Build history of the part. All positions in model axes, mm. Give positions to 0.01 mm unless a question says otherwise; leave off trailing zeros. Write each loop counter-clockwise with the first axis right and the second up, starting at its lowest first coordinate (ties: lowest second). Pieces come first, ordered by that corner, then holes. Notation, with made-up numbers: (57, 60.5) - (89, 60.5) arc R18 cw to (89, 84.5) - close; hole circle Ø4 at (-26.75, 77.5). An arc over 180 degrees is marked (long way). Use one line per item in the form item = value. Start each with the question number.
from build123d import *

# Parameters (mm, degrees)
F1_DEPTH = 400
F3_DEPTH = 25.001
F4_R     = 7.9375
F5_DEPTH = 25.001


with BuildPart() as f1:
    # F0 (on Top) → F1 (new body)
    with BuildSketch(Plane.XY):
        with BuildLine():
            ThreePointArc((12.5, 9.5), (11.62132, 11.62132), (9.5, 12.5))
            Line((9.5, 12.5), (-9.5, 12.5))
            ThreePointArc((-9.5, 12.5), (-11.62132, 11.62132), (-12.5, 9.5))
            Line((-12.5, 9.5), (-12.5, -9.5))
            ThreePointArc((-12.5, -9.5), (-11.62132, -11.62132), (-9.5, -12.5))
            Line((-9.5, -12.5), (9.5, -12.5))
            ThreePointArc((9.5, -12.5), (11.62132, -11.62132), (12.5, -9.5))
            Line((12.5, -9.5), (12.5, 9.5))
        make_face()
        with BuildLine():
            Line((-6.5, 9.5), (6.5, 9.5))
            ThreePointArc((6.5, 9.5), (8.62132, 8.62132), (9.5, 6.5))
            Line((9.5, 6.5), (9.5, -6.5))
            ThreePointArc((9.5, -6.5), (8.62132, -8.62132), (6.5, -9.5))
            Line((6.5, -9.5), (-6.5, -9.5))
            ThreePointArc((-6.5, -9.5), (-8.62132, -8.62132), (-9.5, -6.5))
            Line((-9.5, -6.5), (-9.5, 6.5))
            ThreePointArc((-9.5, 6.5), (-8.62132, 8.62132), (-6.5, 9.5))
        make_face(mode=Mode.SUBTRACT)
    extrude(amount=F1_DEPTH)

    # F2 (on face) → F3 (cut, through all)
    with BuildSketch(Plane(origin=(-12.5, 0, 0), x_dir=(0, -1, 0), z_dir=(-1, 0, 0))):
        with BuildLine():
            ThreePointArc((6, 58), (5.414214, 59.414214), (4, 60))
            Line((4, 60), (-4, 60))
            ThreePointArc((-4, 60), (-5.414214, 59.414214), (-6, 58))
            Line((-6, 58), (-6, 12))
            ThreePointArc((-6, 12), (-5.414214, 10.585786), (-4, 10))
            Line((-4, 10), (4, 10))
            ThreePointArc((4, 10), (5.414214, 10.585786), (6, 12))
            Line((6, 12), (6, 58))
        make_face()
        with BuildLine():
            ThreePointArc((6, 118), (5.414214, 119.414214), (4, 120))
            Line((4, 120), (-4, 120))
            ThreePointArc((-4, 120), (-5.414214, 119.414214), (-6, 118))
            Line((-6, 118), (-6, 72))
            ThreePointArc((-6, 72), (-5.414214, 70.585786), (-4, 70))
            Line((-4, 70), (4, 70))
            ThreePointArc((4, 70), (5.414214, 70.585786), (6, 72))
            Line((6, 72), (6, 118))
        make_face()
    extrude(amount=-F3_DEPTH, mode=Mode.SUBTRACT)

    # F4 (on face) → F5 (cut, through all)
    with BuildSketch(Plane.YZ.offset(12.5)):
        with Locations((0, 381)):
            Circle(F4_R)
    extrude(amount=-F5_DEPTH, mode=Mode.SUBTRACT)


solid = f1.part
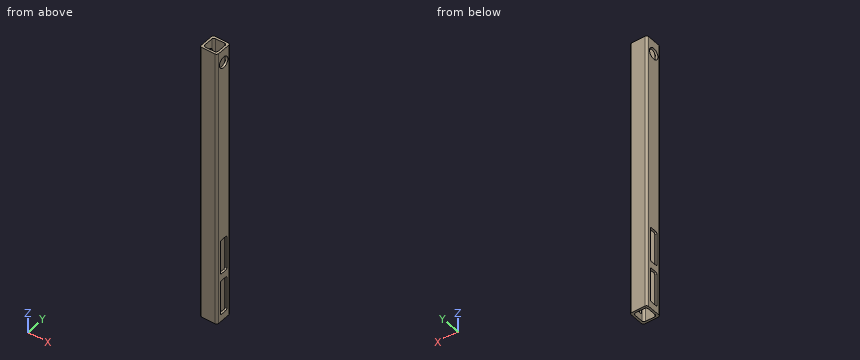
(1) Cut at D-D, the plane z = 76.5. Give the cut face in (x, y).
(2) Wall check: line 1 (Z direction, x = 11.1, y = 0); line 2 (Y direction, x = -1.25, z = 121). Give the ranges that are in metal, low to high. Write a range as from..to.
(3) Cut at B-B, the plane y = 0. State how many separate pieces and enclosed holes the cut face has, then the cut area to 3 significant figures.
(4) Cut at C-C, the plane z = 153. Give the cut face in (x, y).
(5) Cut at A-A, the plane z = 381. Give the cut face in (x, y).
(6) Pin check, flat tips, straight feed: pin 1 Ø2.5 at (x, z) = (11.5, 31) entering from +Y; pin 2 Ø1 at (x, y) = (-2.5, -9.5) entering from -Z; pin 3 Ø3.5 at (x, z) = (11.5, 29) entering from -Y; pin 4 Ø0.9 at (x, z) = (-11.5, 106) entering from -Y. Stop position of each tip, or through.
Solution:
q1.outline = (-12.5, -9.5) arc R3 ccw to (-9.5, -12.5) - (9.5, -12.5) arc R3 ccw to (12.5, -9.5) - (12.5, -6) - (9.5, -6) - (9.5, -6.5) arc R3 cw to (6.5, -9.5) - (-6.5, -9.5) arc R3 cw to (-9.5, -6.5) - (-9.5, -6) - (-12.5, -6) - close; (-12.5, 6) - (-9.5, 6) - (-9.5, 6.5) arc R3 cw to (-6.5, 9.5) - (6.5, 9.5) arc R3 cw to (9.5, 6.5) - (9.5, 6) - (12.5, 6) - (12.5, 9.5) arc R3 ccw to (9.5, 12.5) - (-9.5, 12.5) arc R3 ccw to (-12.5, 9.5) - close
q2.line_1 = 0..10, 60..70, 120..373.06, 388.94..400
q2.line_2 = -12.5..-9.5, 9.5..12.5
q3.separate_pieces = 8
q3.enclosed_holes = 0
q3.area = 1,700 mm2
q4.outline = (-12.5, -9.5) arc R3 ccw to (-9.5, -12.5) - (9.5, -12.5) arc R3 ccw to (12.5, -9.5) - (12.5, 9.5) arc R3 ccw to (9.5, 12.5) - (-9.5, 12.5) arc R3 ccw to (-12.5, 9.5) - close; hole (-9.5, -6.5) arc R3 ccw to (-6.5, -9.5) - (6.5, -9.5) arc R3 ccw to (9.5, -6.5) - (9.5, 6.5) arc R3 ccw to (6.5, 9.5) - (-6.5, 9.5) arc R3 ccw to (-9.5, 6.5) - close
q5.outline = (-12.5, -9.5) arc R3 ccw to (-9.5, -12.5) - (9.5, -12.5) arc R3 ccw to (12.5, -9.5) - (12.5, -7.94) - (9.13, -7.94) arc R3 cw to (6.5, -9.5) - (-6.5, -9.5) arc R3 cw to (-9.13, -7.94) - (-12.5, -7.94) - close; (-12.5, 7.94) - (-9.13, 7.94) arc R3 cw to (-6.5, 9.5) - (6.5, 9.5) arc R3 cw to (9.13, 7.94) - (12.5, 7.94) - (12.5, 9.5) arc R3 ccw to (9.5, 12.5) - (-9.5, 12.5) arc R3 ccw to (-12.5, 9.5) - close
q6.pin_1 = 12.4
q6.pin_2 = 0
q6.pin_3 = -12.49
q6.pin_4 = -12.07
